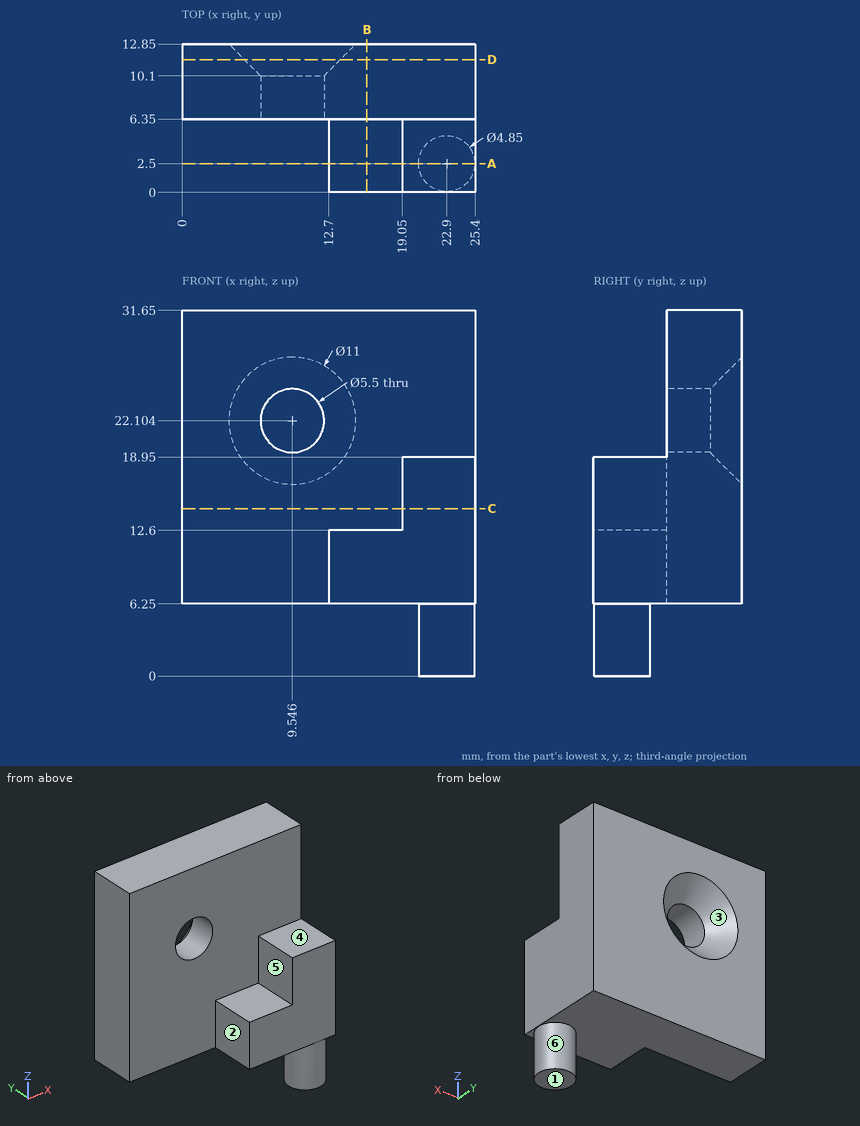
The drawing under review shows one solid part. Ordinate dimensions are in mm from its lowest x, y, z. A direction names the side the tool comes from. Coordinates: 2 decimals unless noted, no trailing zeros. Loops run counter-clockwise (first coordinate to the right, second up) from the corner with the lowest first, then second, coordinate; pieces in that order, holes last.
Item 1: Add section B-B (x = 16). Write out the cut boundary in (y, z).
Completed:
outline: (0, 6.25) - (12.85, 6.25) - (12.85, 31.65) - (6.35, 31.65) - (6.35, 12.6) - (0, 12.6) - close
Item 2: Add section D-D (y = 11.5). Write out the cut boundary in (x, z).
Completed:
outline: (0, 6.25) - (25.4, 6.25) - (25.4, 31.65) - (0, 31.65) - close; hole circle Ø8.3 at (9.55, 22.1)
Item 3: Add section C-C (z = 14.5). Write out the cut boundary in (x, y).
Completed:
outline: (0, 6.35) - (19.05, 6.35) - (19.05, 0) - (25.4, 0) - (25.4, 12.85) - (0, 12.85) - close
Item 4: Add section A-A (y = 2.5). Write out the cut boundary in (x, z) (3 decimals), and give its area (3 significant figures).
Completed:
outline: (12.7, 6.25) - (20.475, 6.25) - (20.475, 0) - (25.325, 0) - (25.325, 6.25) - (25.4, 6.25) - (25.4, 18.95) - (19.05, 18.95) - (19.05, 12.6) - (12.7, 12.6) - close
area: 151 mm2
Item 5: Wall thickness on L1, parallel to Z at x = 22.25, y = 6.25; L2, parallel to Y at x = 10.75, z = 27.5; L3, parallel to Z at x = 18.75, y = 6.75: over which ranges is each line inside the solid? List them lowest first.
Completed:
L1: z = 6.25 to 18.95
L2: y = 6.35 to 12.85
L3: z = 6.25 to 31.65
Item 6: For the marked faces 4, 5 and 6, list the 3-axis set-ups (+Z, -Z, +X, -X, +Y, -Y) from which the entire face can be reached by the end or side of a thin tool; tool diameter is ignored.
Completed:
face 4: +Z, +X, -X, -Y
face 5: +Z, -X, -Y
face 6: -Z
Item 7: Clearance check with flat-ended pins moving along their axes: pin 1 (1 mm diameter, centred on x = 4.5, y = 10, fed in from -Z); pin 2 (3 mm diameter, centred on x = 17.5, y = 1.5, fed in from +Z); pin 3 (1.9 mm diameter, centred on y = 4, z = 17, fed in from -X). State where each tip first meets the part, or that it passes through.
Completed:
pin 1: stops at z = 6.25
pin 2: stops at z = 12.6
pin 3: stops at x = 19.05
Item 8: Draft analysis for pull direction Z (two halves, no side actions). For the marked faces 1, 2 and 3, state which applies: pulls with the +Z half, pulls with the -Z half, needs draft (parallel to the pull), parting line crosses it, or undercut.
Completed:
face 1: pulls with the -Z half
face 2: needs draft
face 3: undercut
